Solid Edge part; units mm, degrees
sketch "Sketch1" plane through (0, 0, 0) normal (0, 0, 1) x (1, 0, 0)
  line L0 (75, 75) -> (-75, 75)
  line L1 (-75, 75) -> (-75, -75)
  line L2 (-75, -75) -> (75, -75)
  line L3 (75, -75) -> (75, 75)
extrude "Protrusion1" add sketch "Sketch1" against normal blind 200
sketch "Sketch2" plane through (0, 0, 0) normal (0, 0, 1) x (1, 0, 0)
  line L0 (147.5, -147.5) -> (147.5, 147.5)
  line L1 (147.5, 147.5) -> (-147.5, 147.5)
  line L2 (-147.5, 147.5) -> (-147.5, -147.5)
  line L3 (-147.5, -147.5) -> (147.5, -147.5)
extrude "VaciadoExtruido_1" cut sketch "Sketch2" against normal blind 195
extrude "VaciadoExtruido_2" [suppressed]
extrude "VaciadoExtruido_3" [suppressed]
sketch "Sketch3" plane through (0, 0, 0) normal (0, 0, 1) x (1, 0, 0)
  line L0 (75, -75) -> (75, 75)
  line L1 (75, 75) -> (-75, 75)
  line L2 (-75, 75) -> (-75, -75)
  line L3 (-75, -75) -> (75, -75)
extrude "ProtrusiónExtruida_2" add sketch "Sketch3" against normal blind 200
sketch "Sketch4" plane through (0, 0, 0) normal (0, 0, 1) x (1, 0, 0)
  line L0 (72.5, -72.5) -> (72.5, 72.5)
  line L1 (72.5, 72.5) -> (-72.5, 72.5)
  line L2 (-72.5, 72.5) -> (-72.5, -72.5)
  line L3 (-72.5, -72.5) -> (72.5, -72.5)
extrude "VaciadoExtruido_4" cut sketch "Sketch4" against normal blind 195
sketch "Sketch5" plane through (75, 0, -100) normal (1, 0, 0) x (0, 1, 0)
  circle A0 centre (0, 50) radius 9
extrude "VaciadoExtruido_5" cut sketch "Sketch5" against normal blind 5
sketch "Sketch6" plane through (75, 0, -100) normal (1, 0, 0) x (0, 1, 0)
  circle A0 centre (0, -25) radius 9
extrude "VaciadoExtruido_6" cut sketch "Sketch6" against normal blind 5
Can you work these out from the model? Positions are in its coordinate system, mm. A direction names the side the tool comes from. Give positions to 0.01 mm unless a question says otherwise; leave off trailing zeros. Order: outer loops, then holes, each group sorted by start corner. A loop starts at its lowest first (then second) coordinate and runs counter-clockwise, first axis right, second up. Notation, with made-up numbers: M -27.5,-22 L 25.5,-22 A21 cw 25.5,17 Z; hole C 80,37 d7. An arc over 180 degrees is marked long. One line per question, with ' | ' between items.
Item 1: I'm going to push flat-ended pins straight in: pin 1 Ø12 at (y, z) = (0.5, -117.5) entering from +X; pin 2 Ø2 at (x, y) = (17, -58.5) entering from +Z. Where does each tip first touch, or does it pass through?
Answer block:
pin 1: stops at x = 75 | pin 2: stops at z = -195
Item 2: We'd pull the mould along Y, two halves only. Please class faces 4 (the face through (75, -1, -99)), 5 (the face through (-1, -75, -99)), 6 (the face through (-72.5, 1, -96)): released by +Y, released by -Y, zero draft, split by the parting line, or undercut.
Answer block:
face 4: zero draft | face 5: released by -Y | face 6: undercut
Item 3: Suppose I cut it at D-D, the plane z = -50. Write out the boundary of the cut face in (x, y).
Answer block:
outline: M -75,-75 L 75,-75 L 75,-9 L 72.5,-9 L 72.5,-72.5 L -72.5,-72.5 L -72.5,72.5 L 72.5,72.5 L 72.5,9 L 75,9 L 75,75 L -75,75 Z
Item 4: Suppose I cut it at B-B, the plane z = -84. Write out the boundary of the cut face in (x, y).
Answer block:
outline: M -75,-75 L 75,-75 L 75,75 L -75,75 Z; hole M -72.5,-72.5 L 72.5,-72.5 L 72.5,72.5 L -72.5,72.5 Z
Item 5: Please list where these lines run through material, in increasing order: L1, parallel to Z at x = 73, y = 0; L2, parallel to Y at x = -42, z = -43.
Answer block:
L1: z = -200 to -134, -116 to -59, -41 to 0 | L2: y = -75 to -72.5, 72.5 to 75
Item 6: For faces 1 (the face through (73.77, -7.14, -130.48)), 2 (the face through (1, 75, -99)), 3 (the face through (1, 72.5, -96)), which set-ups out of +Z, -Z, +X, -X, +Y, -Y let a thin tool reach every point of the face, with its end or its side?
Answer block:
face 1: +X | face 2: +Z, -Z, +X, -X, +Y | face 3: +Z
Item 7: Suppose I cut it at C-C, the plane x = 46. Write out the boundary of the cut face in (y, z), then the cut area to 4 significant figures.
Answer block:
outline: M -75,-200 L 75,-200 L 75,0 L 72.5,0 L 72.5,-195 L -72.5,-195 L -72.5,0 L -75,0 Z | area: 1,725 mm2
Item 8: Suppose I cut it at A-A, the plane y = 0. Write out the boundary of the cut face in (x, z), then the cut area to 4 significant figures.
Answer block:
outline: M -75,-200 L 75,-200 L 75,-134 L 72.5,-134 L 72.5,-195 L -72.5,-195 L -72.5,0 L -75,0 Z; M 72.5,-116 L 75,-116 L 75,-59 L 72.5,-59 Z; M 72.5,-41 L 75,-41 L 75,0 L 72.5,0 Z | area: 1,635 mm2
